Geometry: see drawing. Coordinates: mm, zero at the bounding-box minimum. A direction names the side the tool comes from. Give positions to 0.01 mm unless a question says otherwise; leave off trailing zeros. Write each loop counter-clockwise with the first axis right and the second up, starting at its lowest first coordinate (ties: lowest second). Pieces come first, ordered by that corner, then holes. Notation, with made-up numbers: (50.25, 43.5) - (106.25, 43.5) arc R34 ccw to (106.25, 77.5) - close; hole circle Ø7 at (74.5, 55.5). An arc over 180 degrees is marked (long way). Answer as CSV lines item,"result". Start each with the question number.
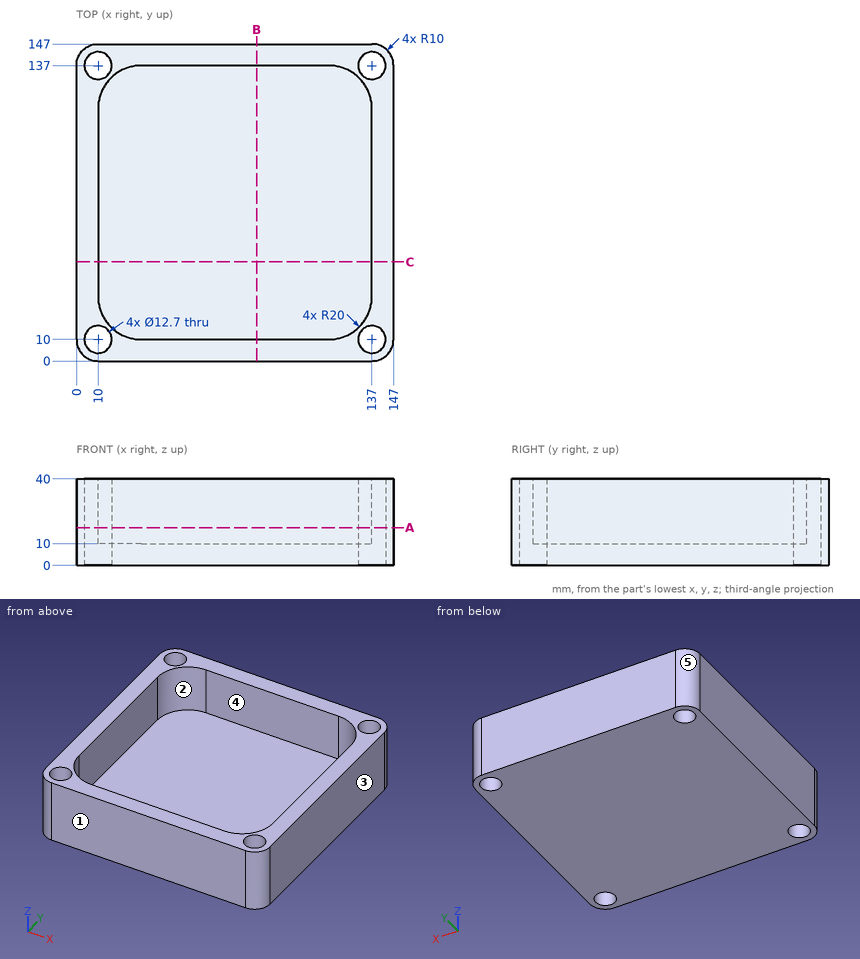
1) Material intervals for line 1 (X direction, y = 102, z = 26.5); line 2 (X direction, y = 8.5, z = 18); line 3 (Y direction, x = 139, z = 7.5), sorted ascending. Write a range as from..to.
2) Pull-direction query (Y, two-part tool) for the marked faces 1, 2 and 3; classes: +Y half, -Y half, draft (parallel to the pull), parting line (faces both ways), or undercut.
3) Contact query for flat-ended pins moving along their axis: P1, Ø7.5, axis at x = 10, y = 10, coming from the -Z side; P2, Ø20.5, axis at x = 137, y = 10, coming from the -Z side; P3, Ø1, axis at x = 39, y = 78.5, coming from the +Z side. Output: stop coordinate, or through.
4) Reachability of the marked faces 4 and 5 from +Z, -Z, +X, -X, +Y, -Y: full face, straight path, thin tool, end or side. Return the list, or none.
5) Cut plane B-B on x = 83.5. Output: boundary loops of the cut face in (y, z), and give its area (3 significant figures).
6) Cut plane A-A on z = 17.5. Output: boundary loops of the cut face in (x, y).
Numbers:
1,line 1,"x = 0..10, 137..147"
1,line 2,"x = 0.11..3.83, 16.17..130.83, 143.17..146.89"
1,line 3,"y = 0.2..3.97, 16.03..130.97, 143.03..146.8"
2,face 1,"-Y half"
2,face 2,"undercut"
2,face 3,"draft"
3,P1,"passes through"
3,P2,"stops at z = 0"
3,P3,"stops at z = 10"
4,face 4,"+Z"
4,face 5,"+Z, -Z, -X, +Y"
5,outline,"(0, 0) - (147, 0) - (147, 40) - (137, 40) - (137, 10) - (10, 10) - (10, 40) - (0, 40) - close"
5,area,"2,070 mm²"
6,outline,"(0, 10) arc R10 ccw to (10, 0) - (137, 0) arc R10 ccw to (147, 10) - (147, 137) arc R10 ccw to (137, 147) - (10, 147) arc R10 ccw to (0, 137) - close; hole circle Ø12.7 at (10, 10); hole circle Ø12.7 at (10, 137); hole (10, 30) arc R20 ccw to (30, 10) - (117, 10) arc R20 ccw to (137, 30) - (137, 117) arc R20 ccw to (117, 137) - (30, 137) arc R20 ccw to (10, 117) - close; hole circle Ø12.7 at (137, 10); hole circle Ø12.7 at (137, 137)"
